from build123d import *

# Parameters (mm, degrees)
ESQUISSE1_W             = 15
ESQUISSE1_H             = 5.05
BOSS_EXTRU_1_DEPTH      = 3
ESQUISSE2_R             = 7.5
ESQUISSE2_R_2           = 1.6
ENL_V_MAT_EXTRU_1_DEPTH = 37.18010503
ESQUISSE3_R             = 1.5
ENL_V_MAT_EXTRU_2_DEPTH = 37.18010503


with BuildPart() as part:
    # Esquisse1 → Boss.-Extru.1 (new body)
    with BuildSketch(Plane.XY):
        with BuildLine():
            Line((-20, 20), (20, 20))
            ThreePointArc((20, 20), (27.071067812, 17.071067812), (30, 10))
            Line((30, 10), (30, -20))
            Line((30, -20), (-30, -20))
            Line((-30, -20), (-30, 10))
            ThreePointArc((-30, 10), (-27.071067812, 17.071067812), (-20, 20))
        make_face()
        with Locations((15, -14)):
            Rectangle(ESQUISSE1_W, ESQUISSE1_H, mode=Mode.SUBTRACT)
        with Locations((-15, -14)):
            Rectangle(ESQUISSE1_W, ESQUISSE1_H, mode=Mode.SUBTRACT)
    extrude(amount=BOSS_EXTRU_1_DEPTH)

    # Esquisse2 → Enlèv. mat.-Extru.1 (cut, through all)
    with BuildSketch(Plane.XY.offset(3)):
        with Locations((11, -35.28215794)):
            Circle(ESQUISSE2_R)
        with Locations((-11, 3.753166138)):
            Circle(ESQUISSE2_R_2)
    extrude(amount=-ENL_V_MAT_EXTRU_1_DEPTH, mode=Mode.SUBTRACT)

    # Esquisse3 → Enlèv. mat.-Extru.2 (cut, through all)
    with BuildSketch(Plane(origin=(0, 0, 0), x_dir=(-1, 0, 0), z_dir=(0, 0, -1))):
        with Locations((-25.75, 8.753166138)):
            Circle(ESQUISSE3_R)
        with Locations((-25.75, -1.246833862)):
            Circle(ESQUISSE3_R)
        with Locations((23.75, 8.753166138)):
            Circle(ESQUISSE3_R)
        with Locations((23.75, -1.246833862)):
            Circle(ESQUISSE3_R)
    extrude(amount=-ENL_V_MAT_EXTRU_2_DEPTH, mode=Mode.SUBTRACT)


solid = part.part
Read the model definition and answer for the solid it produces. Units are mm, in the model's axes. A direction names the side the tool comes from. Coordinates: 2 decimals unless noted, no trailing zeros. Order: outer loops, then holes, each group sorted by start corner. A loop starts at its lowest first (then second) coordinate and runs counter-clockwise, first axis right, second up. Notation, with made-up numbers: (-38, 75) -> (-1, 75) arc R22 ccw to (-1, 87) -> close; hole circle Ø2 at (59, -37). An arc over 180 degrees is marked (long way). Answer as a JSON object with one key per item and string values.
1) A cutting plane is placed at D-D, the plane x = 25.75. Determine the outline of the cut face in (y, z).
Model answer:
{"outline": "(-20, 0) -> (-2.75, 0) -> (-2.75, 3) -> (-20, 3) -> close; (0.25, 0) -> (7.25, 0) -> (7.25, 3) -> (0.25, 3) -> close; (10.25, 0) -> (18.18, 0) -> (18.18, 3) -> (10.25, 3) -> close"}
2) The mould has two halves that part along Y. Classify faces 1 (the face through (22.5, -14, 1)), 2 (the face through (0, -20, 1)), 3 (the face through (0, 0, 3)): released by +Y, released by -Y, zero draft, split by the parting line, or undercut.
Model answer:
{"face 1": "undercut", "face 2": "released by -Y", "face 3": "zero draft"}
3) A cutting plane is placed at C-C, the plane z = 1.4. Determine the outline of the cut face in (x, y) (3 decimals).
Model answer:
{"outline": "(-30, -20) -> (30, -20) -> (30, 10) arc R10 ccw to (20, 20) -> (-20, 20) arc R10 ccw to (-30, 10) -> close; hole circle Ø3 at (-23.75, -1.247); hole circle Ø3 at (-23.75, 8.753); hole (-22.5, -16.525) -> (-7.5, -16.525) -> (-7.5, -11.475) -> (-22.5, -11.475) -> close; hole circle Ø3.2 at (-11, 3.753); hole (7.5, -16.525) -> (22.5, -16.525) -> (22.5, -11.475) -> (7.5, -11.475) -> close; hole circle Ø3 at (25.75, -1.247); hole circle Ø3 at (25.75, 8.753)"}
4) Consider line 1 along Y through (x, z) = (-11, 1.2) (3 decimals); line 2 along X through (y, z) = (-12.5, 2.6); line 3 along Y through (x, z) = (13, 2.4) (3 decimals). Determine where each line is inside the solid, lowest interval first. Write a range as from..to.
Model answer:
{"line 1": "y = -20..-16.525, -11.475..2.153, 5.353..20", "line 2": "x = -30..-22.5, -7.5..7.5, 22.5..30", "line 3": "y = -20..-16.525, -11.475..20"}
5) A tool of negligible diameter and unlimited length cuts with its end or side. For faces 4 (the face through (-15, -11.475, 1)), 5 (the face through (0, 20, 1)), from which of +Z, -Z, +X, -X, +Y, -Y can it reach the whole face along a straight path? Write none if from no direction.
Model answer:
{"face 4": "+Z, -Z", "face 5": "+Z, -Z, +X, -X, +Y"}
6) A cutting plane is placed at B-B, the plane x = -11. Determine the outline of the cut face in (y, z) (3 decimals), plus the area to 4 significant figures.
Model answer:
{"outline": "(-20, 0) -> (-16.525, 0) -> (-16.525, 3) -> (-20, 3) -> close; (-11.475, 0) -> (2.153, 0) -> (2.153, 3) -> (-11.475, 3) -> close; (5.353, 0) -> (20, 0) -> (20, 3) -> (5.353, 3) -> close", "area": "95.25 mm²"}
7) A cutting plane is placed at A-A, the plane x = 16. Determine the outline of the cut face in (y, z) (3 decimals).
Model answer:
{"outline": "(-20, 0) -> (-16.525, 0) -> (-16.525, 3) -> (-20, 3) -> close; (-11.475, 0) -> (20, 0) -> (20, 3) -> (-11.475, 3) -> close"}
